from build123d import *

# Parameters (mm, degrees)
CROQUIS1_W              = 666
CROQUIS1_H              = 300
SALIENTE_EXTRUIR1_DEPTH = 1.5
CROQUIS2_W              = 24
CROQUIS2_H              = 46.5
CORTAR_EXTRUIR1_DEPTH   = 2.5
CROQUIS3_W              = 38
CROQUIS3_H              = 14
CORTAR_EXTRUIR2_DEPTH   = 2.5
CROQUIS5_W              = 24
CROQUIS5_H              = 30
CORTAR_EXTRUIR3_DEPTH   = 2.5


with BuildPart() as part:
    # Croquis1 → Saliente-Extruir1 (new body)
    with BuildSketch(Plane(origin=(0, 0, 0), x_dir=(1, 0, 0), z_dir=(0, 1, 0))):
        Rectangle(CROQUIS1_W, CROQUIS1_H)
    extrude(amount=SALIENTE_EXTRUIR1_DEPTH)

    # Croquis2 → Cortar-Extruir1 (cut, through all)
    with BuildSketch(Plane(origin=(0, 1.5, 0), x_dir=(1, 0, 0), z_dir=(0, 1, 0))):
        with Locations((321, 126.75)):
            Rectangle(CROQUIS2_W, CROQUIS2_H)
        with Locations((-321, 126.75)):
            Rectangle(CROQUIS2_W, CROQUIS2_H)
        with Locations((-321, -126.75)):
            Rectangle(CROQUIS2_W, CROQUIS2_H)
        with Locations((321, -126.75)):
            Rectangle(CROQUIS2_W, CROQUIS2_H)
    extrude(amount=-CORTAR_EXTRUIR1_DEPTH, mode=Mode.SUBTRACT)

    # Croquis3 → Cortar-Extruir2 (cut, through all)
    with BuildSketch(Plane(origin=(0, 1.5, 0), x_dir=(1, 0, 0), z_dir=(0, 1, 0))):
        with Locations((-290, 143)):
            Rectangle(CROQUIS3_W, CROQUIS3_H)
        with Locations((290, 143)):
            Rectangle(CROQUIS3_W, CROQUIS3_H)
        with Locations((290, -143)):
            Rectangle(CROQUIS3_W, CROQUIS3_H)
        with Locations((-290, -143)):
            Rectangle(CROQUIS3_W, CROQUIS3_H)
    extrude(amount=-CORTAR_EXTRUIR2_DEPTH, mode=Mode.SUBTRACT)

    # Croquis5 → Cortar-Extruir3 (cut, through all)
    with BuildSketch(Plane(origin=(0, 1.5, 0), x_dir=(1, 0, 0), z_dir=(0, 1, 0))):
        with Locations((-321, 88.5)):
            Rectangle(CROQUIS5_W, CROQUIS5_H)
        with Locations((321, 88.5)):
            Rectangle(CROQUIS5_W, CROQUIS5_H)
        with Locations((321, -88.5)):
            Rectangle(CROQUIS5_W, CROQUIS5_H)
        with Locations((-321, -88.5)):
            Rectangle(CROQUIS5_W, CROQUIS5_H)
    extrude(amount=-CORTAR_EXTRUIR3_DEPTH, mode=Mode.SUBTRACT)


solid = part.part
Input: part model. Units: mm. Frame: model coordinates. Give positions to 0.01 mm unless a question says otherwise; leave off trailing zeros. Order: outer loops, then holes, each group sorted by start corner. A loop starts at its lowest first (then second) coordinate and runs counter-clockwise, first axis right, second up. Notation, with made-up numbers: M -14.5,35.25 L -7.5,35.25 A8 ccw -7.5,47.25 Z; hole C 72.25,76.5 d1. An arc over 180 degrees is marked long. Answer as a JSON object with one key per item and string values.
1. Cut plane A-A, the plane y = 1.05. Output: boundary loops of the cut face in (x, z).
Result sheet:
{"outline": "M -333,-73.5 L -309,-73.5 L -309,-136 L -271,-136 L -271,-150 L 271,-150 L 271,-136 L 309,-136 L 309,-73.5 L 333,-73.5 L 333,73.5 L 309,73.5 L 309,136 L 271,136 L 271,150 L -271,150 L -271,136 L -309,136 L -309,73.5 L -333,73.5 Z"}
2. Ray query, line 1 (X direction, y = 0.55, z = 109). Return the intervals inside material, ascending. Write a range as [from, to].
Result sheet:
{"line 1": "[-309, 309]"}
3. Cut plane B-B, the plane z = -101. Output: boundary loops of the cut face in (x, y).
Result sheet:
{"outline": "M -309,0 L 309,0 L 309,1.5 L -309,1.5 Z"}
4. First-contact query: P1, Ø0.8, axis at x = 297, y = 1, coming from the -Z side; P2, Ø0.8, axis at x = 321, y = 1, coming from the +Z side. Flat tips, straight axial feed; report the tip coordinate or a pass-through.
Result sheet:
{"P1": "z = -136", "P2": "z = 73.5"}
